from build123d import *

# Parameters (mm, degrees)
SKETCH1_W           = 8
SKETCH1_H           = 50
BOSS_EXTRUDE1_DEPTH = 8


with BuildPart() as part:
    # Sketch1 → Boss-Extrude1 (new body)
    with BuildSketch(Plane(origin=(0, 0, 0), x_dir=(1, 0, 0), z_dir=(0, 1, 0))):
        with Locations((-4, 44.105)):
            Rectangle(SKETCH1_W, SKETCH1_H)
        Polygon((110, 0), (110, 88.21), (0, 88.21), (0, 69.105), (0, 19.105), (0, 0), align=None)
        Polygon((220, 88.21), (110, 88.21), (110, 0), (220, 0), (220, 19.105), (220, 69.105), align=None)
        with Locations((224, 44.105)):
            Rectangle(SKETCH1_W, SKETCH1_H)
    extrude(amount=BOSS_EXTRUDE1_DEPTH)


solid = part.part
Design review of the part built by this model. Coordinates are the model's own, in mm. A direction names the side the tool comes from. Round coordinates to 2 decimals unless told otherwise and drop trailing zeros. Write each loop counter-clockwise with the first axis right and the second up, starting at its lowest first coordinate (ties: lowest second). Pieces come first, ordered by that corner, then holes. Notation, with made-up numbers: (75, -32) - (127, -32) arc R21 ccw to (127, -8) - close; hole circle Ø1 at (85, 30.25). An arc over 180 degrees is marked (long way). Return JSON: item names as keys, results as strings. Group by question number.
Item 1: Machinability: for faces 1 (the face through (224, 4, -69.105)), 2 (the face through (220, 4, -9)), 3 (the face through (-4, 4, -69.105)), 4 (the face through (0, 4, -10)), which of the approach directions +Z, -Z, +X, -X, +Y, -Y give a long, thin tool a straight path to every point of the face, cutting with its end or side? Answer none if there is none.
Item 2: We need section B-B on z = -77.5. Write out the cut boundary in (x, y), and give its area (3 significant figures).
Item 3: Insertion check: P1, Ø3, axis at x = 99, z = -9, coming from the -Y side; P2, Ø4, axis at y = 3.5, z = -9.5, coming from the -X side; P3, Ø2.5, axis at y = 3, z = -79.5, coming from the +X side; P4, Ø4, axis at x = -4.5, y = 3.5, coming from the -Z side (3 decimals). Each pin has a flat end and moves straight along its axis. Give the tip position at first contact, or say it passes through.
Item 4: We need section A-A on y = 2.5. Write out the cut boundary in (x, z) (3 decimals), and give its area (3 significant figures).
Item 5: For probe 1 along X at (y, z) = (3, -70), list the stretches that pass through material, from the lowest coordinate up. Write a range as [from, to].
Model answer:
{
 "1": {"face 1": "-Z, +X, +Y, -Y", "face 2": "+Z, +X, +Y, -Y", "face 3": "-Z, -X, +Y, -Y", "face 4": "+Z, -X, +Y, -Y"},
 "2": {"outline": "(0, 0) - (220, 0) - (220, 8) - (0, 8) - close", "area": "1,760 mm²"},
 "3": {"P1": "stops at y = 0", "P2": "stops at x = 0", "P3": "stops at x = 220", "P4": "stops at z = -69.105"},
 "4": {"outline": "(-8, -69.105) - (0, -69.105) - (0, -88.21) - (220, -88.21) - (220, -69.105) - (228, -69.105) - (228, -19.105) - (220, -19.105) - (220, 0) - (0, 0) - (0, -19.105) - (-8, -19.105) - close", "area": "20,200 mm²"},
 "5": {"probe 1": "x = [0, 220]"}
}
